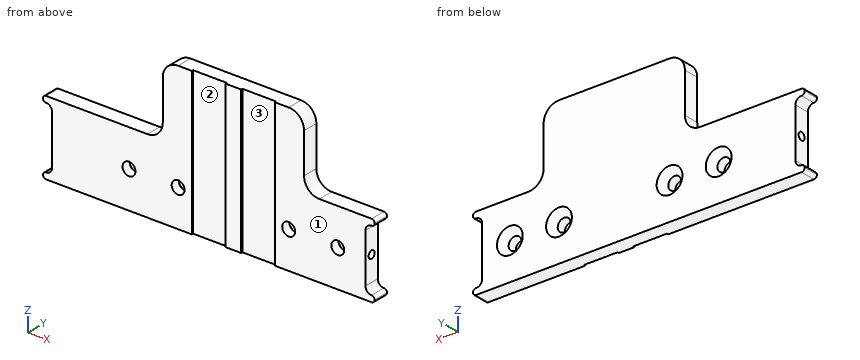
Autodesk Inventor part; units mm, degrees
ref_plane "Arbeitsebene1" through (-51, 0, 12) normal (0, 0, -1) x (-1, 0, 0)
ref_plane "YZ Plane" through (0, 0, 0) normal (1, 0, 0) x (0, 1, 0)
ref_plane "XZ Plane" through (0, 0, 0) normal (0, 1, 0) x (-1, 0, 0)
sketch "Skizze1" plane through (0, 0, 0) normal (0, 1, 0) x (-1, 0, 0)
  line L0 (-54, 0) -> (54, 0)
  line L1 (54, 0) -> (54, 24)
  line L2 (54, 24) -> (15, 24)
  line L3 (15, 24) -> (15, 47)
  line L4 (15, 47) -> (-31, 47)
  line L5 (-31, 47) -> (-31, 24)
  line L6 (-31, 24) -> (-54, 24)
  line L7 (-54, 24) -> (-54, 0)
  point P0 (0, 0)
  point P1 (0, 0)
  dimension "d0" = 108
  dimension "d1" = 24
  dimension "d2" = 39
  dimension "d3" = 23
  dimension "d59" = 23
extrude "Extrusion1" add sketch "Skizze1" along normal blind 5
sketch "Skizze2" plane through (54, 0, 24) normal (1, 0, 0) x (0, 0, -1)
  line L0 (0, 0) -> (24, 0)
  line L1 (24, 0) -> (24, 5)
  line L2 (0, 5) -> (24, 5)
  line L3 (0, 0) -> (0, 5)
  line L4 (2, 0) -> (22, 0)
  line L5 (22, 0) -> (22, 5)
  line L6 (22, 5) -> (2, 5)
  line L7 (2, 5) -> (2, 0)
  dimension "d7" = 2
  dimension "d8" = 2
extrude "Extrusion2" cut sketch "Skizze2" against normal blind 3 contours L7 L2 L5 L0
sketch "Skizze3" plane through (-54, 0, 0) normal (-1, 0, 0) x (0, 0, 1)
  line L0 (0, 0) -> (24, 0)
  line L1 (24, 0) -> (24, 5)
  line L2 (0, 5) -> (24, 5)
  line L3 (0, 0) -> (0, 5)
  line L4 (2, 0) -> (22, 0)
  line L5 (22, 0) -> (22, 5)
  line L6 (22, 5) -> (2, 5)
  line L7 (2, 5) -> (2, 0)
  dimension "d11" = 2
  dimension "d12" = 2
extrude "Extrusion3" cut sketch "Skizze3" against normal blind 3 contours L7 L2 L5 L0
fillet "Rundung1" radius 1 8 edges at (-54, 2.5, 0) (-54, 2.5, 2) (-54, 2.5, 22) (-54, 2.5, 24) (54, 2.5, 24) (54, 2.5, 22) (54, 2.5, 2) (54, 2.5, 0)
fillet "Rundung2" radius 5 4 edges at (31, 2.5, 24) (31, 2.5, 47) (-15, 2.5, 47) (-15, 2.5, 24)
sketch "Skizze4" plane through (53, 0, 0) normal (0, 0, -1) x (-1, 0, 0)
  line L0 (58.5, -0.5) -> (47.5, -0.5)
  line L1 (47.5, -0.5) -> (47.5, 0.5)
  line L2 (47.5, 0.5) -> (58.5, 0.5)
  line L3 (58.5, 0.5) -> (58.5, -0.5)
  line L4 (58.5, -0.5) -> (47.5, 0.5) construction
  line L5 (47.5, -0.5) -> (58.5, 0.5) construction
  point P0 (53, 0)
  dimension "d17" = 11
  dimension "d18" = 1
extrude "Extrusion4" cut sketch "Skizze4" against normal through all
sketch "Skizze6" plane through (0, 5, 0) normal (0, 1, 0) x (1, 0, 0)
  line L0 (53, 0) -> (-53, 0)
  point P0 (0, 0)
  point P1 (-26, -12)
  point P2 (26, -12)
  dimension "d31" = 12
  dimension "d32" = 26
  dimension "d33" = 26
hole "Bohrung2" at (-26, 5, 12) at (26, 5, 12) direction (0, -1, 0) diameter 4.2 end through all countersink diameter 8.4 countersink angle 90
sketch "Skizze7" plane through (51, 0, 24) normal (1, 0, 0) x (0, 0, -1)
  line L0 (22, 5) -> (22, 0)
  line L1 (2, 5) -> (22, 5)
  point P0 (24, 0)
  point P1 (12, 2.5)
  dimension "d41" = 2.5
  dimension "d42" = 10
hole "Bohrung3" at (51, 2.5, 12) direction (-1, 0, 0) diameter 2.459 depth 6 tip angle 118
sketch "Skizze8" plane through (-51, 0, 0) normal (-1, 0, 0) x (0, 0, 1)
  line L0 (2, 5) -> (22, 5)
  line L1 (2, 0) -> (2, 5)
  point P0 (0, 0)
  point P1 (12, 2.5)
  dimension "d50" = 2.5
  dimension "d51" = 10
hole "Bohrung4" at (-51, 2.5, 12) direction (1, 0, 0) diameter 2.459 depth 6 tip angle 118
ref_plane "Arbeitsebene1" through (-51, 0, 12) normal (0, 0, -1) x (-1, 0, 0)
pattern_linear "Rechteckige Anordnung1" count 2 spacing 16 along (1, 0, 0) of "Extrusion4", "Bohrung2"
fillet "Rundung3" radius 2 4 edges at (51, 2.5, 22) (51, 2.5, 2) (-51, 2.5, 22) (-51, 2.5, 2)
properties part number "GrundplatteeThumbloop"
Check sheet for the modelled part. Datum: model origin and axes. Units: mm. Face numbers are marked on the shaded views. Round coordinates to 2 decimals unless told otherwise and drop trailing zeros. Order: outer loops, then holes, each group sorted by start corner. A loop starts at its lowest first (then second) coordinate and runs counter-clockwise, first axis right, second up.
1) Scan lines: line 1 (X direction, y = 1.15, z = 12); line 2 (Y direction, x = 47.05, z = 12); line 3 (Z direction, x = 46.5, y = 2.5). Record each from-to range of solid material in increasing order.
2) Go/stop test with flat-tipped pins: pin 1 Ø0.6 at (y, z) = (0.5, 12) entering from +X; pin 2 Ø1.5 at (y, z) = (2.5, 37) entering from -X; pin 3 Ø3 at (x, y) = (-14.5, 1) entering from -Z; pin 4 Ø5.5 at (x, z) = (26, 12) entering from +Y. Record where each tip stops, or that it passes through.
3) Section check A-A (x = -26). Record the boundary of the cut face in (y, z), and give its area (3 significant figures).
4) Section check C-C (z = 6). Record the boundary of the cut face in (x, y).
5) Mould release check, pull along X, two halves, no side actions. Record for the marked faces 1, 2 and 3: +X half, -X half, draft (parallel to the pull), parting line (faces both ways), or undercut.
6) Section check B-B (z = 37.5). Record the boundary of the cut face in (x, y).
Result:
1. line 1: x = -51 to -28.1, -23.9 to -12.1, -7.9 to 23.9, 28.1 to 39.9, 44.1 to 51
1. line 2: y = 0 to 1.27, 3.73 to 5
1. line 3: z = 0 to 10.77, 13.23 to 24
2. pin 1: stops at x = 51
2. pin 2: stops at x = -15
2. pin 3: stops at z = 0
2. pin 4: stops at y = 3.55
3. outline: (0, 0) - (5, 0) - (5, 7.8) - (2.9, 9.9) - (0, 9.9) - close; (0, 14.1) - (2.9, 14.1) - (5, 16.2) - (5, 24) - (0, 24) - close
3. area: 94.6 mm2
4. outline: (-51, 0) - (-5.5, 0) - (-5.5, 0.5) - (5.5, 0.5) - (5.5, 0) - (10.5, 0) - (10.5, 0.5) - (21.5, 0.5) - (21.5, 0) - (51, 0) - (51, 5) - (-51, 5) - close
5. face 1: draft
5. face 2: undercut
5. face 3: undercut
6. outline: (-15, 0) - (-5.5, 0) - (-5.5, 0.5) - (5.5, 0.5) - (5.5, 0) - (10.5, 0) - (10.5, 0.5) - (21.5, 0.5) - (21.5, 0) - (31, 0) - (31, 5) - (-15, 5) - close
